```python
from build123d import *

# Parameters (mm, degrees)
SKETCH1_W           = 120
SKETCH1_H           = 400
BOSS_EXTRUDE1_DEPTH = 3
CUT_EXTRUDE1_DEPTH  = 3
SKETCH3_R           = 2
CUT_EXTRUDE2_DEPTH  = 3
SKETCH4_W           = 120
SKETCH4_H           = 44
CUT_EXTRUDE3_DEPTH  = 10
SKETCH5_R           = 2
CUT_EXTRUDE4_DEPTH  = 10


with BuildPart() as part:
    # Sketch1 → Boss-Extrude1 (new body)
    with BuildSketch(Plane.XY):
        Rectangle(SKETCH1_W, SKETCH1_H)
    extrude(amount=BOSS_EXTRUDE1_DEPTH)

    # Sketch2 → Cut-Extrude1 (cut)
    with BuildSketch(Plane.XY.offset(3)):
        with BuildLine():
            Line((-35.5, -116), (35.5, -116))
            ThreePointArc((35.5, -116), (37.621320344, -116.878679656), (38.5, -119))
            Line((38.5, -119), (38.5, -156))
            ThreePointArc((38.5, -156), (37.621320344, -158.121320344), (35.5, -159))
            Line((35.5, -159), (-35.5, -159))
            ThreePointArc((-35.5, -159), (-37.621320344, -158.121320344), (-38.5, -156))
            Line((-38.5, -156), (-38.5, -119))
            ThreePointArc((-38.5, -119), (-37.621320344, -116.878679656), (-35.5, -116))
        make_face()
        with BuildLine():
            Line((-35.5, 84), (35.5, 84))
            ThreePointArc((35.5, 84), (37.621320344, 83.121320344), (38.5, 81))
            Line((38.5, 81), (38.5, 44))
            ThreePointArc((38.5, 44), (37.621320344, 41.878679656), (35.5, 41))
            Line((35.5, 41), (-35.5, 41))
            ThreePointArc((-35.5, 41), (-37.621320344, 41.878679656), (-38.5, 44))
            Line((-38.5, 44), (-38.5, 81))
            ThreePointArc((-38.5, 81), (-37.621320344, 83.121320344), (-35.5, 84))
        make_face()
    extrude(amount=-CUT_EXTRUDE1_DEPTH, mode=Mode.SUBTRACT)

    # Sketch3 → Cut-Extrude2 (cut)
    with BuildSketch(Plane.XY.offset(3)):
        with Locations((-30, 185)):
            Circle(SKETCH3_R)
        with Locations((-30, 65)):
            Circle(SKETCH3_R)
        with Locations((-30, -55)):
            Circle(SKETCH3_R)
        with Locations((-30, -175)):
            Circle(SKETCH3_R)
        with Locations(Location((30, -175, 0), (0, 0, 180))):
            Circle(SKETCH3_R)
        with Locations(Location((30, -55, 0), (0, 0, 180))):
            Circle(SKETCH3_R)
        with Locations((30, 65)):
            Circle(SKETCH3_R)
        with Locations(Location((30, 185, 0), (0, 0, 180))):
            Circle(SKETCH3_R)
    extrude(amount=-CUT_EXTRUDE2_DEPTH, mode=Mode.SUBTRACT)

    # Sketch4 → Cut-Extrude3 (cut)
    with BuildSketch(Plane.XY.offset(3)):
        with Locations((0, -178)):
            Rectangle(SKETCH4_W, SKETCH4_H)
    extrude(amount=-CUT_EXTRUDE3_DEPTH, mode=Mode.SUBTRACT)

    # Sketch5 → Cut-Extrude4 (cut)
    with BuildSketch(Plane.XY.offset(3)):
        with Locations((-28, -108)):
            Circle(SKETCH5_R)
        with Locations((28, -108)):
            Circle(SKETCH5_R)
    extrude(amount=-CUT_EXTRUDE4_DEPTH, mode=Mode.SUBTRACT)


solid = part.part
```
For this review, take the finished solid that the model builds, in its own axes (mm). Coordinates: 2 decimals unless noted, no trailing zeros. Write each loop counter-clockwise with the first axis right and the second up, starting at its lowest first coordinate (ties: lowest second). Pieces come first, ordered by that corner, then holes.
(1) Add section A-A on x = 21.5. Give the boundary of the cut face in (y, z), then the cut area to 3 significant figures.
(2) Wall thickness on probe 1 along X at (y, z) = (185, 2.25); probe 2 along Y at (x, z) = (25.5, 2.45); probe 3 along X at (y, z) = (68, 2.7): over which ranges is each line inside the solid? List them lowest first.
(3) For pin 1 Ø2.5 at (x, y) = (-28, -108) entering from +Z (3 decimals); pin 2 Ø0.9 at (x, z) = (16, 1) entering from -Y, all flat-tipped, find the tip position at first contact; note any pin that passes through.
(4) Add section B-B on z = 0.7. Give the boundary of the cut face in (x, y), then the cut area to 3 significant figures.
Answer sheet:
1. outline: (-116, 0) - (41, 0) - (41, 3) - (-116, 3) - close; (84, 0) - (200, 0) - (200, 3) - (84, 3) - close
1. area: 819 mm2
2. probe 1: x = -60 to -32, -28 to 28, 32 to 60
2. probe 2: y = -116 to 41, 84 to 200
2. probe 3: x = -60 to -38.5, 38.5 to 60
3. pin 1: passes through
3. pin 2: stops at y = -116
4. outline: (-60, -156) - (-38.5, -156) - (-38.5, -119) arc R3 cw to (-35.5, -116) - (35.5, -116) arc R3 cw to (38.5, -119) - (38.5, -156) - (60, -156) - (60, 200) - (-60, 200) - close; hole (-38.5, 44) arc R3 ccw to (-35.5, 41) - (35.5, 41) arc R3 ccw to (38.5, 44) - (38.5, 81) arc R3 ccw to (35.5, 84) - (-35.5, 84) arc R3 ccw to (-38.5, 81) - close; hole circle Ø4 at (-30, -55); hole circle Ø4 at (-30, 185); hole circle Ø4 at (-28, -108); hole circle Ø4 at (28, -108); hole circle Ø4 at (30, -55); hole circle Ø4 at (30, 185)
4. area: 36,300 mm2
